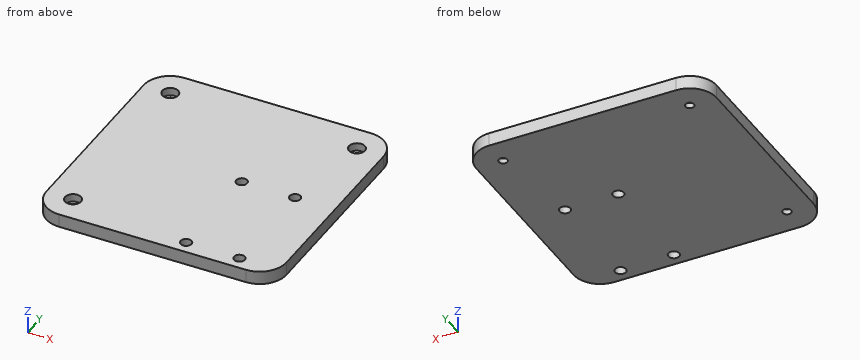
```python
from build123d import *

# Parameters (mm, degrees)
SKETCH_1_R          = 1.6
EXTRUDE_1_DEPTH     = 5
SKETCH_2_R          = 3
CUT_EXTRUDE_1_DEPTH = 3
SKETCH_3_R          = 2.05
CUT_EXTRUDE_2_DEPTH = 64.835726674


with BuildPart() as part:
    # ｽｹｯﾁ1 → ﾎﾞｽ - 押し出し1 (new body)
    with BuildSketch(Plane.XY):
        with BuildLine():
            Line((-35, 45), (35, 45))
            ThreePointArc((35, 45), (42.071067812, 42.071067812), (45, 35))
            Line((45, 35), (45, -35))
            ThreePointArc((45, -35), (42.071067812, -42.071067812), (35, -45))
            Line((35, -45), (-35, -45))
            ThreePointArc((-35, -45), (-42.071067812, -42.071067812), (-45, -35))
            Line((-45, -35), (-45, 35))
            ThreePointArc((-45, 35), (-42.071067812, 42.071067812), (-35, 45))
        make_face()
        with Locations((-35, -35)):
            Circle(SKETCH_1_R, mode=Mode.SUBTRACT)
        with Locations((-35, 35)):
            Circle(SKETCH_1_R, mode=Mode.SUBTRACT)
        with Locations((35, 35)):
            Circle(SKETCH_1_R, mode=Mode.SUBTRACT)
    extrude(amount=EXTRUDE_1_DEPTH)

    # ｽｹｯﾁ2 → ｶｯﾄ - 押し出し1 (cut)
    with BuildSketch(Plane.XY.offset(5)):
        with Locations((-35, 35)):
            Circle(SKETCH_2_R)
        with Locations((35, 35)):
            Circle(SKETCH_2_R)
        with Locations((-35, -35)):
            Circle(SKETCH_2_R)
    extrude(amount=-CUT_EXTRUDE_1_DEPTH, mode=Mode.SUBTRACT)

    # ｽｹｯﾁ3 → ｶｯﾄ - 押し出し2 (cut, through all)
    with BuildSketch(Plane.XY.offset(5)):
        with Locations((30, 0)):
            Circle(SKETCH_3_R)
        with Locations((10, 0)):
            Circle(SKETCH_3_R)
        with Locations((10, -40)):
            Circle(SKETCH_3_R)
        with Locations((30, -40)):
            Circle(SKETCH_3_R)
    extrude(amount=-CUT_EXTRUDE_2_DEPTH, mode=Mode.SUBTRACT)


solid = part.part
```
Verification items for the finished model (mm, model axes). Round coordinates to 2 decimals unless told otherwise and drop trailing zeros. Order: outer loops, then holes, each group sorted by start corner. A loop starts at its lowest first (then second) coordinate and runs counter-clockwise, first axis right, second up. Notation, with made-up numbers: (41, 52.25) -> (75, 52.25) arc R18 cw to (75, 79.25) -> close; hole circle Ø1 at (-7.75, -5). An arc over 180 degrees is marked (long way). Put each result on its own line as item: value. Start each with the question number.
(1) Section check A-A (y = 0). Enter the section's corners in (x, z), then the cut area to 3 significant figures.
(2) Section check C-C (z = 1.05). Enter the section's corners in (x, y).
(3) Section check B-B (x = 10). Enter the section's corners in (y, z).
(4) Material ranges on line 1 along Y through (x, z) = (-35, 1.3); line 2 along Y through (x, z) = (35, 3.3), recorded low to high.
(5) Depth check by flat-ended pin: pin 1 Ø3 at (x, y) = (-35.5, 35.5) entering from +Z. Enter the tip coordinate at first touch or a pass-through.
Completed:
1. outline: (-45, 0) -> (7.95, 0) -> (7.95, 5) -> (-45, 5) -> close; (12.05, 0) -> (27.95, 0) -> (27.95, 5) -> (12.05, 5) -> close; (32.05, 0) -> (45, 0) -> (45, 5) -> (32.05, 5) -> close
1. area: 409 mm2
2. outline: (-45, -35) arc R10 ccw to (-35, -45) -> (35, -45) arc R10 ccw to (45, -35) -> (45, 35) arc R10 ccw to (35, 45) -> (-35, 45) arc R10 ccw to (-45, 35) -> close; hole circle Ø3.2 at (-35, -35); hole circle Ø3.2 at (-35, 35); hole circle Ø4.1 at (10, -40); hole circle Ø4.1 at (10, 0); hole circle Ø4.1 at (30, -40); hole circle Ø4.1 at (30, 0); hole circle Ø3.2 at (35, 35)
3. outline: (-45, 0) -> (-42.05, 0) -> (-42.05, 5) -> (-45, 5) -> close; (-37.95, 0) -> (-2.05, 0) -> (-2.05, 5) -> (-37.95, 5) -> close; (2.05, 0) -> (45, 0) -> (45, 5) -> (2.05, 5) -> close
4. line 1: y = -45 to -36.6, -33.4 to 33.4, 36.6 to 45
4. line 2: y = -45 to 32, 38 to 45
5. pin 1: stops at z = 2
